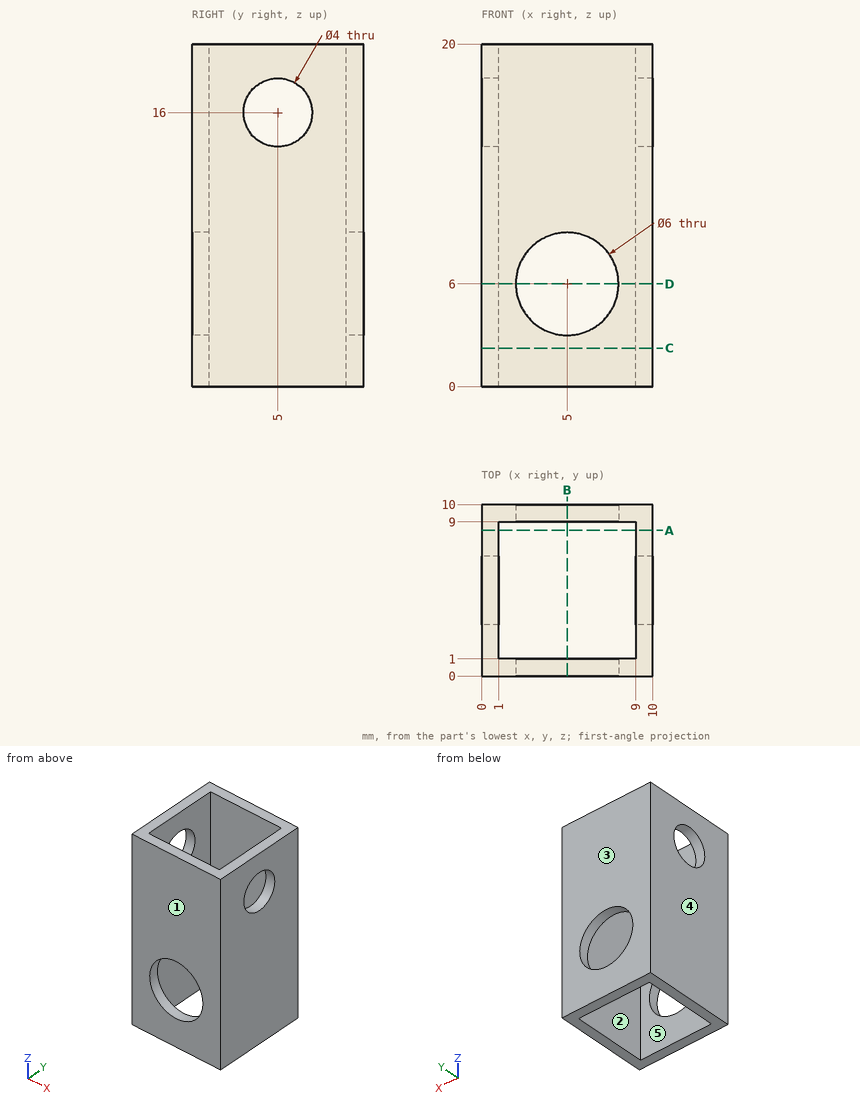
Part print with two shaded views. Sizes in mm from the minimum x, y, z corner. A direction names the side the tool comes from. Round coordinates to 2 decimals unless told otherwise and drop trailing zeros. Write each loop counter-clockwise with the first axis right and the second up, starting at its lowest first coordinate (ties: lowest second). Pieces come first, ordered by that corner, then holes. Notation, with made-up numbers: M -8.5,43.5 L 20.5,43.5 A14 ccw 20.5,68.5 Z; hole C -26.5,-1.75 d11. An arc over 180 degrees is marked long. Put each result on its own line as item: value. Start each with the question number.
1) Pull direction Y, two halves, no side cores. Call the marked faces 3, 4 and 5: pulls with the +Y half, pulls with the -Y half, needs draft (parallel to the pull), parting line crosses it, or undercut.
2) Saw through at B-B, the plane x = 5. Write the cut outline in (y, z), and give its area (3 significant figures).
3) Saw through at D-D, the plane z = 6. Write the cut outline in (x, y), and give its area (3 significant figures).
4) Saw through at A-A, the plane y = 8.5. Write the cut outline in (x, z).
5) 3-axis set-ups, long thin cutter, end or side, ignore diameter. For the marked faces 1 and 2: which of +Z, -Z, +X, -X, +Y, -Y reach the whole face in a straight line?
6) Saw through at C-C, the plane z = 2.25. Write the cut outline in (x, y), and give its area (3 significant figures).
7) Drill centre lines: probe 1 along X at (y, z) = (2, 6.25); probe 2 along Z at (x, y) = (0.5, 5). Where is each one in solid material? Low to high. Write a range as [from, to].
Resolved:
1. face 3: pulls with the +Y half
1. face 4: needs draft
1. face 5: undercut
2. outline: M 0,0 L 1,0 L 1,3 L 0,3 Z; M 0,9 L 1,9 L 1,20 L 0,20 Z; M 9,0 L 10,0 L 10,3 L 9,3 Z; M 9,9 L 10,9 L 10,20 L 9,20 Z
2. area: 28.0 mm²
3. outline: M 0,0 L 2,0 L 2,1 L 1,1 L 1,9 L 2,9 L 2,10 L 0,10 Z; M 8,0 L 10,0 L 10,10 L 8,10 L 8,9 L 9,9 L 9,1 L 8,1 Z
3. area: 24.0 mm²
4. outline: M 0,0 L 1,0 L 1,20 L 0,20 Z; M 9,0 L 10,0 L 10,20 L 9,20 Z
5. face 1: +Z, -Z, +X, -X, -Y
5. face 2: +Z, -Z
6. outline: M 0,0 L 10,0 L 10,10 L 0,10 Z; hole M 1,1 L 9,1 L 9,9 L 1,9 Z
6. area: 36.0 mm²
7. probe 1: [0, 1], [9, 10]
7. probe 2: [0, 14], [18, 20]
